Model file for the job. Use its own axes, mm. A direction names the side the tool comes from. Coordinates: 2 decimals unless noted, no trailing zeros. Write each loop counter-clockwise with the first axis right and the second up, starting at its lowest first coordinate (ties: lowest second). Pieces come first, ordered by that corner, then holes. Notation, with made-up numbers: (16, 0.5) - (31, 0.5) arc R10 ccw to (31, 10.5) - close; hole circle Ø6 at (60, 5). An arc over 180 degrees is marked (long way). Put each result on its own line as item: value. Start each with the question number.
1. Drop flat-ended pins along their axis: P1, Ø10, axis at x = -12, z = 61.5, coming from the -Y side; P2, Ø2.5, axis at y = 1, z = 127.5, coming from the -X side; P3, Ø1, axis at y = 67.5, z = 99.5, coming from the +X side. Give the stop position or say it passes through.
2. Saw through at D-D, the plane z = 33.5. Write the cut outline in (x, y), plus the area to 3 significant figures.
3. Saw through at B-B, the plane x = 0. Write the cut outline in (y, z) (3 decimals), plus the area to 3 significant figures.
4. Pull direction Z, two halves, no side cores. Call faces 4 (the face through (76.962, 35, 127)), 5 (the face through (24, 70, 133.35)), 6 (the face through (-74.6, 1.5, 123.99)): released by +Z, released by -Z, zero draft, split by the parting line, or undercut.
5. Saw through at C-C, the plane x = -74. Write the cut outline in (y, z) (3 decimals), plus the area to 3 significant figures.
6. Drill centre lines: L1, parallel to Z at x = 74, y = 2 (3 decimals); L2, parallel to Y at x = 23.5, z = 80.5; L3, parallel to X at y = 9, z = 122.5. Where is each one in solid material? Low to high. Write a range as from..to.
7. Which spindle directions (+Z, -Z, +X, -X, +Y, -Y) get a long thin tool onto all of the face, cutting with end or side? Do faces 1 (the face through (-7, 72.39, 59)), 2 (the face through (-71, 3.048, 6)), 3 (the face through (-78, 29, 12.192)). Say none if no direction does.
8. Saw through at A-A, the plane y = 27. Write the cut outline in (x, z), plus the area to 3 significant figures.
```python
from build123d import *

# Parameters (mm, degrees)
BOSS_EXTRU_1_DEPTH      = 133.35
ESQUISSE3_W             = 108.966
ESQUISSE3_H             = 68.58
ENL_V_MAT_EXTRU_1_DEPTH = 222.799600766
CONG_1_R                = 2.54
CONG_2_R                = 2.54
ESQUISSE6_R             = 10
ENL_V_MAT_EXTRU_4_DEPTH = 174.176969023
ESQUISSE9_R             = 16
ENL_V_MAT_EXTRU_5_DEPTH = 3.81
SKETCH1_R               = 2.75
CUT_EXTRUDE1_DEPTH      = 3.048


with BuildPart() as part:
    # Esquisse2 → Boss.-Extru.1 (new body)
    with BuildSketch(Plane.XY):
        Polygon((-64.77, 0), (-80.01, 0), (-80.01, 76.2), (80.01, 76.2), (80.01, 0), (64.77, 0), (64.77, 3.048), (76.962, 3.048), (76.962, 68.58), (-76.962, 68.58), (-76.962, 3.048), (-64.77, 3.048), align=None)
    extrude(amount=BOSS_EXTRU_1_DEPTH)

    # Esquisse3 → Enlèv. mat.-Extru.1 (cut, through all)
    with BuildSketch(Plane.ZY.offset(80.01)):
        with Locations((66.675, 34.29)):
            Rectangle(ESQUISSE3_W, ESQUISSE3_H)
    extrude(amount=-ENL_V_MAT_EXTRU_1_DEPTH, mode=Mode.SUBTRACT)

    # Congé1
    cong_1_edges = [part.edges().sort_by_distance(p)[0] for p in [
        (-80.01, 0, 127.254),
        (80.01, 0, 127.254),
        (-80.01, 0, 6.096),
        (80.01, 0, 6.096),
    ]]
    fillet(cong_1_edges, radius=CONG_1_R)

    # Congé2
    cong_2_edges = [part.edges().sort_by_distance(p)[0] for p in [
        (0, 76.2, 0),
        (-80.01, 76.2, 66.675),
        (80.01, 76.2, 66.675),
        (0, 76.2, 133.35),
    ]]
    fillet(cong_2_edges, radius=CONG_2_R)

    # Esquisse6 → Enlèv. mat.-Extru.4 (cut, through all)
    with BuildSketch(Plane(origin=(0, 76.2, 0), x_dir=(1, 0, 0), z_dir=(0, 1, 0))):
        with Locations(Location((0, -66.675, 0), (0, 0, 270))):
            Circle(ESQUISSE6_R)
    extrude(amount=-ENL_V_MAT_EXTRU_4_DEPTH, mode=Mode.SUBTRACT)

    # Esquisse9 → Enlèv. mat.-Extru.5 (cut)
    with BuildSketch(Plane(origin=(0, 76.2, 0), x_dir=(1, 0, 0), z_dir=(0, 1, 0))):
        with Locations(Location((0, -66.675, 0), (0, 0, 270))):
            Circle(ESQUISSE9_R)
    extrude(amount=-ENL_V_MAT_EXTRU_5_DEPTH, mode=Mode.SUBTRACT)

    # Sketch1 → Cut-Extrude1 (cut)
    with BuildSketch(Plane.XZ):
        with Locations((74, 126.675)):
            Circle(SKETCH1_R)
        with Locations((74, 6.675)):
            Circle(SKETCH1_R)
        with Locations((-74, 6.675)):
            Circle(SKETCH1_R)
        with Locations((-74, 126.675)):
            Circle(SKETCH1_R)
    extrude(amount=-CUT_EXTRUDE1_DEPTH, mode=Mode.SUBTRACT)


solid = part.part
```
Final values:
1. P1: stops at y = 68.58
1. P2: stops at x = -79.99
1. P3: passes through
2. outline: (-80.01, 68.58) - (80.01, 68.58) - (80.01, 73.66) arc R2.54 ccw to (77.47, 76.2) - (-77.47, 76.2) arc R2.54 ccw to (-80.01, 73.66) - close
2. area: 1,220 mm²
3. outline: (68.58, 0) - (73.66, 0) arc R2.54 ccw to (76.2, 2.54) - (76.2, 50.675) - (72.39, 50.675) - (72.39, 56.675) - (68.58, 56.675) - close; (68.58, 76.675) - (72.39, 76.675) - (72.39, 82.675) - (76.2, 82.675) - (76.2, 130.81) arc R2.54 ccw to (73.66, 133.35) - (68.58, 133.35) - close
3. area: 815 mm²
4. face 4: zero draft
4. face 5: released by +Z
4. face 6: undercut
5. outline: (0, 0) - (3.048, 0) - (3.048, 3.925) - (0, 3.925) - close; (0, 9.425) - (3.048, 9.425) - (3.048, 12.192) - (0, 12.192) - close; (0, 121.158) - (3.048, 121.158) - (3.048, 123.925) - (0, 123.925) - close; (0, 129.425) - (3.048, 129.425) - (3.048, 133.35) - (0, 133.35) - close; (68.58, 0) - (73.66, 0) arc R2.54 ccw to (76.2, 2.54) - (76.2, 130.81) arc R2.54 ccw to (73.66, 133.35) - (68.58, 133.35) - close
5. area: 1,050 mm²
6. L1: z = 0..3.925, 9.425..12.192, 121.158..123.925, 129.425..133.35
6. L2: y = 68.58..76.2
6. L3: x = -80.01..-76.96, 76.96..80.01
7. face 1: +Y
7. face 2: +Z, -Z
7. face 3: +X, -X, -Y
8. outline: (-80.01, 0) - (-76.96, 0) - (-76.96, 12.19) - (-80.01, 12.19) - close; (-80.01, 121.16) - (-76.96, 121.16) - (-76.96, 133.35) - (-80.01, 133.35) - close; (76.96, 0) - (80.01, 0) - (80.01, 12.19) - (76.96, 12.19) - close; (76.96, 121.16) - (80.01, 121.16) - (80.01, 133.35) - (76.96, 133.35) - close
8. area: 149 mm²
